Here's how the part is built. I have some questions about the finished solid (model axes, mm). Face numbers are marked on the shaded views. A direction names the side the tool comes from. Give positions to 0.01 mm unless a question says otherwise; leave off trailing zeros. Write each loop counter-clockwise with the first axis right and the second up, starting at its lowest first coordinate (ties: lowest second). Pieces come first, ordered by that corner, then holes. Notation, with made-up numbers: M 20,51 L 28,51 A18 ccw 28,55 Z; hole C -18,-9 d11. An arc over 180 degrees is marked long. Use one line per item in the form item = value. Start each with the question number.
from build123d import *

# Parameters (mm, degrees)
SKETCH1_R                       = 2.5
BOSS_EXTRUDE1_DEPTH             = 24
SKETCH2_R                       = 11
BOSS_EXTRUDE2_DEPTH             = 2
SKETCH3_W                       = 41.5
SKETCH3_H                       = 41.5
BOSS_EXTRUDE3_DEPTH             = 40
CUT_EXTRUDE1_DEPTH              = 71.40685336
CUT_EXTRUDE1_DEPTH_BACK         = 71.40685336
M3X0_5_TAPPED_HOLE1_D           = 2.5
M3X0_5_TAPPED_HOLE1_DEPTH       = 7.5
M3X0_5_TAPPED_HOLE1_CBORE_D     = 3
M3X0_5_TAPPED_HOLE1_CBORE_DEPTH = 6
M3X0_5_TAPPED_HOLE1_TIP         = 0.751075774
CUT_EXTRUDE2_START              = -15
CUT_EXTRUDE2_DEPTH              = 15
CUT_EXTRUDE3_DEPTH              = 10.5


with BuildPart() as part:
    # Sketch1 → Boss-Extrude1 (new body)
    with BuildSketch(Plane.XY):
        Circle(SKETCH1_R)
    extrude(amount=BOSS_EXTRUDE1_DEPTH)

    # Sketch2 → Boss-Extrude2 (add)
    with BuildSketch(Plane(origin=(0, 0, 0), x_dir=(-1, 0, 0), z_dir=(0, 0, -1))):
        Circle(SKETCH2_R)
    extrude(amount=-BOSS_EXTRUDE2_DEPTH)

    # Sketch3 → Boss-Extrude3 (add)
    with BuildSketch(Plane(origin=(0, 0, 0), x_dir=(-1, 0, 0), z_dir=(0, 0, -1))):
        Rectangle(SKETCH3_W, SKETCH3_H)
    extrude(amount=BOSS_EXTRUDE3_DEPTH)

    # Sketch4 → Cut-Extrude1 (cut, two sides: drawn at the far end of the back side and taken through both)
    with BuildSketch(Plane(origin=(0, 0, -40), x_dir=(-1, 0, 0), z_dir=(0, 0, -1)).offset(-CUT_EXTRUDE1_DEPTH_BACK)):
        with BuildLine():
            Line((-20.75, -16.482945732), (-20.75, -20.75))
            Line((-20.75, -20.75), (-16.482945732, -20.75))
            ThreePointArc((-16.482945732, -20.75), (-18.738329701, -18.738329701), (-20.75, -16.482945732))
        make_face()
        with BuildLine():
            Line((16.482945732, -20.75), (20.75, -20.75))
            Line((20.75, -20.75), (20.75, -16.482945732))
            ThreePointArc((20.75, -16.482945732), (18.738329701, -18.738329701), (16.482945732, -20.75))
        make_face()
        with BuildLine():
            Line((20.75, 16.482945732), (20.75, 20.75))
            Line((20.75, 20.75), (16.482945732, 20.75))
            ThreePointArc((16.482945732, 20.75), (18.738329701, 18.738329701), (20.75, 16.482945732))
        make_face()
        with BuildLine():
            Line((-16.482945732, 20.75), (-20.75, 20.75))
            Line((-20.75, 20.75), (-20.75, 16.482945732))
            ThreePointArc((-20.75, 16.482945732), (-18.738329701, 18.738329701), (-16.482945732, 20.75))
        make_face()
    extrude(amount=CUT_EXTRUDE1_DEPTH + CUT_EXTRUDE1_DEPTH_BACK, mode=Mode.SUBTRACT)

    # M3x0.5 Tapped Hole1
    with Locations(Plane.XY):
        with Locations((-15.5, 15.5), (-15.5, -15.5), (15.5, -15.5), (15.5, 15.5)):
            CounterBoreHole(M3X0_5_TAPPED_HOLE1_D / 2, M3X0_5_TAPPED_HOLE1_CBORE_D / 2, M3X0_5_TAPPED_HOLE1_CBORE_DEPTH, depth=M3X0_5_TAPPED_HOLE1_DEPTH)
            with Locations((0, 0, -(M3X0_5_TAPPED_HOLE1_DEPTH + M3X0_5_TAPPED_HOLE1_TIP / 2))):  # 118° drill point
                Cone(0, M3X0_5_TAPPED_HOLE1_D / 2, M3X0_5_TAPPED_HOLE1_TIP, mode=Mode.SUBTRACT)

    # Sketch7 → Cut-Extrude2 (cut)
    with BuildSketch(Plane.XY.offset(24).offset(CUT_EXTRUDE2_START)):
        with BuildLine():
            Line((-1.5, 2), (1.5, 2))
            ThreePointArc((1.5, 2), (0, 2.5), (-1.5, 2))
        make_face()
    extrude(amount=CUT_EXTRUDE2_DEPTH, mode=Mode.SUBTRACT)

    # Sketch8 → Cut-Extrude3 (cut, symmetric)
    with BuildSketch(Plane.XY.offset(-24)):
        with BuildLine():
            Line((16.482945732, 20.75), (-16.482945732, 20.75))
            ThreePointArc((-16.482945732, 20.75), (-18.738329701, 18.738329701), (-20.75, 16.482945732))
            Line((-20.75, 16.482945732), (-20.75, -16.482945732))
            ThreePointArc((-20.75, -16.482945732), (-18.738329701, -18.738329701), (-16.482945732, -20.75))
            Line((-16.482945732, -20.75), (16.482945732, -20.75))
            ThreePointArc((16.482945732, -20.75), (18.738329701, -18.738329701), (20.75, -16.482945732))
            Line((20.75, -16.482945732), (20.75, 16.482945732))
            ThreePointArc((20.75, 16.482945732), (18.738329701, 18.738329701), (16.482945732, 20.75))
        make_face()
        with BuildLine():
            Line((-14.091752907, 20.65), (14.091752907, 20.65))
            ThreePointArc((14.091752907, 20.65), (17.67766953, 17.67766953), (20.65, 14.091752907))
            Line((20.65, 14.091752907), (20.65, -14.091752907))
            ThreePointArc((20.65, -14.091752907), (17.67766953, -17.67766953), (14.091752907, -20.65))
            Line((14.091752907, -20.65), (-14.091752907, -20.65))
            ThreePointArc((-14.091752907, -20.65), (-17.67766953, -17.67766953), (-20.65, -14.091752907))
            Line((-20.65, -14.091752907), (-20.65, 14.091752907))
            ThreePointArc((-20.65, 14.091752907), (-17.67766953, 17.67766953), (-14.091752907, 20.65))
        make_face(mode=Mode.SUBTRACT)
    extrude(amount=CUT_EXTRUDE3_DEPTH, both=True, mode=Mode.SUBTRACT)


solid = part.part
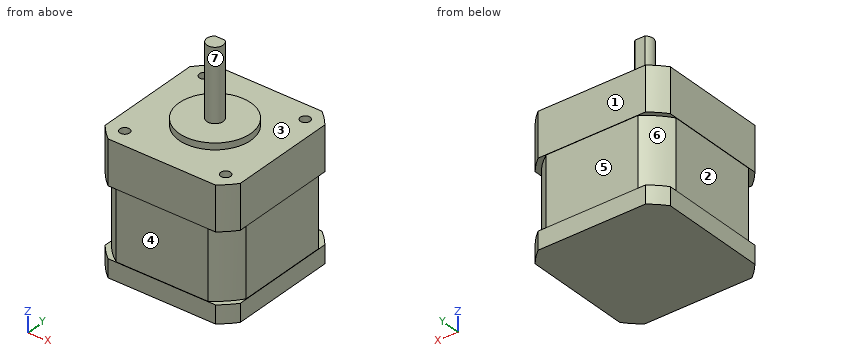
1) Suppose I cut it at B-B, the plane z = -12. List the corners of the cut face in (x, y) for me, and give its area (3 significant figures).
2) On a 3-axis mill with a long thin cutter (end or side, diameter ignored), from which of +Z, -Z, +X, -X, +Y, -Y can I reach the whole of each face in a straight line? I mean the marked faces 4, 5, 6 and 7. Say none if no direction works.
3) Will these pins go through, and if not, where does the flat tip stop? P1, Ø2, axis at y = -0.5, z = -33, coming from the -X side; P2, Ø12, axis at y = 12, z = -20.5, coming from the +X side; P3, Ø2.5, axis at x = 0.5, z = 19, coming from the +Y side.
4) Suppose I cut it at D-D, the plane x = 0. List the corners of the cut face in (y, z) for me, and give its area (3 significant figures).
5) Thinking about a two-plate mould opening in Z: for the marked faces 1, 2 and 3, which applies, released by +Z, released by -Z, zero draft, split by the parting line, or undercut?
6) Suppose I cut it at A-A, the plane z = -2. List the corners of the cut face in (x, y) for me.
7) Please list where these lines run through material, in increasing order: line 1 (Y direction, x = -15.5, z = -1.95); line 2 (X direction, y = -15.5, z = -6.8).
8) Suppose I cut it at C-C, the plane y = 13. List the corners of the cut face in (x, z) for me, and give its area (3 significant figures).
Checks:
q1.outline = M -20.75,-16.48 A26.5 ccw -16.48,-20.75 L 16.48,-20.75 A26.5 ccw 20.75,-16.48 L 20.75,16.48 A26.5 ccw 16.48,20.75 L -16.48,20.75 A26.5 ccw -20.75,16.48 Z
q1.area = 1,690 mm^2
q2.face_4 = +X, -X, -Y
q2.face_5 = +X, -X, +Y
q2.face_6 = -X, +Y
q2.face_7 = +Z
q3.P1 = -20.65
q3.P2 = 20.65
q3.P3 = 2
q4.outline = M -20.75,-40 L 20.75,-40 L 20.75,-34.5 L 20.65,-34.5 L 20.65,-13.5 L 20.75,-13.5 L 20.75,0 L 11,0 L 11,2 L 2.5,2 L 2.5,9 L 2,9 L 2,24 L -2.5,24 L -2.5,2 L -11,2 L -11,0 L -20.75,0 L -20.75,-13.5 L -20.65,-13.5 L -20.65,-34.5 L -20.75,-34.5 Z
q4.area = 1,800 mm^2
q5.face_1 = zero draft
q5.face_2 = undercut
q5.face_3 = released by +Z
q6.outline = M -20.75,-16.48 A26.5 ccw -16.48,-20.75 L 16.48,-20.75 A26.5 ccw 20.75,-16.48 L 20.75,16.48 A26.5 ccw 16.48,20.75 L -16.48,20.75 A26.5 ccw -20.75,16.48 Z; hole C -15.5,-15.5 d3; hole C -15.5,15.5 d3; hole C 15.5,-15.5 d3; hole C 15.5,15.5 d3
q7.line_1 = -20.75 to -17, -14 to 14, 17 to 20.75
q7.line_2 = -20.75 to -16.75, -14.25 to 14.25, 16.75 to 20.75
q8.outline = M -20.75,-40 L 20.75,-40 L 20.75,-34.5 L 20.65,-34.5 L 20.65,-13.5 L 20.75,-13.5 L 20.75,0 L -20.75,0 L -20.75,-13.5 L -20.65,-13.5 L -20.65,-34.5 L -20.75,-34.5 Z
q8.area = 1,660 mm^2
